Source: CAD feature listing. Evaluate the final solid. Frame: model axes, mm. A direction names the side the tool comes from. Round coordinates to 2 decimals unless told otherwise and drop trailing zeros. Write each loop counter-clockwise with the first axis right and the second up, starting at its lowest first coordinate (ties: lowest second). Pieces come first, ordered by that corner, then holes. Notation, with made-up numbers: M 67.5,77 L 93.5,77 A19 ccw 93.5,98 Z; hole C -10,13.25 d6. An arc over 180 degrees is marked long. Answer in a Markdown table with one row per item.
from build123d import *

# Parameters (mm, degrees)
STOCK_TOP_1_START                              = 44.45
STOCK_TOP_1_OUTLINE_W                          = 44.45
STOCK_TOP_1_OUTLINE_H                          = 60.96
STOCK_TOP_1_DEPTH                              = 2.54
STOCK_TOP_1_START_2                            = 43.942
STOCK_TOP_1_2_OUTLINE_W                        = 44.45
STOCK_TOP_1_2_OUTLINE_H                        = 60.96
STOCK_TOP_1_2_DEPTH                            = 0.508
OUTSIDE_FILLET_R                               = 2.54
CUT_A_BIT_OF_THE_ENCLOSURE_REACH               = 48.789
SKETCH1_W                                      = 1.334667882
SKETCH1_H                                      = 23.182275167
SKETCH2_W                                      = 3.81
SKETCH2_H                                      = 7.62
BATTERY_LID_1_DEPTH                            = 19.05
SKETCH3_W                                      = 2.54
SKETCH3_H                                      = 2.54
BATTERY_LID_HOLE_1_DEPTH                       = 1.778
CUT_EXTRUDE1_REACH                             = 64.264
SKETCH5_W                                      = 2.54
SKETCH5_H                                      = 2.54
BATTERY_LID_HOLE_2_DEPTH                       = 1.778
CUT_EXTRUDE2_REACH                             = 64.264
DETACH_LID_ATTACHEMENTS_REACH                  = 52.124
SKETCH9_W                                      = 1.524
SKETCH9_H                                      = 7.62
REMOVE_THE_INNARDS_OF_THE_LID_ATTACHMENT_DEPTH = 19.812
SKETCH11_W                                     = 1.167614697
SKETCH11_H                                     = 1.542617542
SKETCH11_W_2                                   = 1.626626063
SKETCH11_H_2                                   = 1.11023807
BOSS_EXTRUDE4_DEPTH                            = 1.778


# Read off the part's stored shape, not the designer's step: Stock-Top-1
with BuildPart() as part:
    # Stock-Top-1 outline → Stock-Top-1 (new body)
    with BuildSketch(Plane(origin=(0, 0, 0), x_dir=(1, 0, 0), z_dir=(0, 1, 0)).offset(STOCK_TOP_1_START)):
        with Locations((-1.821227893, 7.677651333)):
            Rectangle(STOCK_TOP_1_OUTLINE_W, STOCK_TOP_1_OUTLINE_H)
    extrude(amount=STOCK_TOP_1_DEPTH)

    # Stock-Top-1 2 outline → Stock-Top-1 2 (add)
    with BuildSketch(Plane(origin=(0, 0, 0), x_dir=(1, 0, 0), z_dir=(0, 1, 0)).offset(STOCK_TOP_1_START_2)):
        with Locations((-1.821227893, 7.677651333)):
            Rectangle(STOCK_TOP_1_2_OUTLINE_W, STOCK_TOP_1_2_OUTLINE_H)
        Polygon((11.494723241, -11.994444065), (17.863772107, -11.994444065), (17.863772107, -20.262348667), (-21.506227893, -20.262348667), (-21.506227893, -11.994444065), (-15.225663022, -11.994444065), (-15.225663022, 35.617651333), (11.494723241, 35.617651333), align=None, mode=Mode.SUBTRACT)
    extrude(amount=STOCK_TOP_1_2_DEPTH)

    # Enclosure: sweep along a path in Outline of Enclosure
    with BuildLine(Plane.XZ.offset(-43.942)) as enclosure_path:
        Line((-24.046227893, 22.802348667), (-24.046227893, -38.157651333))
        Line((-24.046227893, -38.157651333), (20.403772107, -38.157651333))
        Line((20.403772107, -38.157651333), (20.403772107, 22.802348667))
        Line((20.403772107, 22.802348667), (-24.046227893, 22.802348667))
    # Shape of Enclosure → Enclosure (sweep)
    with BuildSketch(Plane(origin=(20.403772107, 0, 0), x_dir=(0, 0, -1), z_dir=(1, 0, 0))):
        Polygon((38.157651333, 44.429907846), (38.442131333, 44.429907846), (38.442131333, 40.688820131), (39.070756728, 40.688820131), (39.070756728, 45.242521161), (38.157651333, 45.242521161), align=None)
    sweep(path=enclosure_path.line, transition=Transition.RIGHT)

    # Outside Fillet
    # the kernel refuses this fillet: 2.54 mm, written as the material it takes off along each edge
    with BuildSketch(Plane(origin=(20.403772107, 46.99, 28.835336218), x_dir=(2.8274047493178717e-10, -1.0, 0), z_dir=(0, 0, -1))) as outside_fillet_piece_1:
        with BuildLine():
            CenterArc((2.539999999, 2.413195021), OUTSIDE_FILLET_R, 180.000000016, 71.819221529)
            Line((-1e-09, 2.41319502), (-0.050800001, 2.41319502))
            Line((-0.050800001, 2.41319502), (-0.0508, 0))
            Line((-0.0508, 0), (0, -0.0508))
            ThreePointArc((0, -0.0508), (0.873739419, -0.0508), (1.731628415, -0.0482639))
            Line((1.731628415, -0.0482639), (1.747478839, 0))
        make_face()
    extrude(amount=73.025975102, mode=Mode.SUBTRACT)
    with BuildSketch(Plane(origin=(-24.046227893, 46.99, -44.190638886), x_dir=(2.827486071359672e-10, -1.0, 0), z_dir=(0, 0, 1))) as outside_fillet_piece_2:
        with BuildLine():
            CenterArc((2.540000001, 2.413195021), OUTSIDE_FILLET_R, 179.999999984, 71.819221529)
            Line((1e-09, 2.413195021), (-0.050799999, 2.413195021))
            Line((-0.050799999, 2.413195021), (-0.0508, 0))
            Line((-0.0508, 0), (0, -0.0508))
            ThreePointArc((0, -0.0508), (0.873739419, -0.0508), (1.731628415, -0.0482639))
            Line((1.731628415, -0.0482639), (1.747478839, 0))
        make_face()
    extrude(amount=73.025975107, mode=Mode.SUBTRACT)
    with BuildSketch(Plane(origin=(-30.079215446, 46.99, 22.802348667), x_dir=(0, -1.0, -1.349945893887387e-10), z_dir=(1, 0, 0))) as outside_fillet_piece_3:
        with BuildLine():
            CenterArc((2.54, 2.413195021), OUTSIDE_FILLET_R, 179.999999992, 71.819221529)
            Line((0, 2.413195021), (-0.0508, 2.413195021))
            Line((-0.0508, 2.413195021), (-0.0508, 0))
            Line((-0.0508, 0), (0, -0.0508))
            ThreePointArc((0, -0.0508), (0.873739419, -0.0508), (1.731628415, -0.0482639))
            Line((1.731628415, -0.0482639), (1.747478839, 0))
        make_face()
    extrude(amount=56.515975105, mode=Mode.SUBTRACT)
    with BuildSketch(Plane(origin=(26.436759659, 46.99, -38.157651333), x_dir=(0, 0, 1), z_dir=(-1, 0, 0))) as outside_fillet_piece_4:
        with BuildLine():
            CenterArc((2.413195021, -2.54), OUTSIDE_FILLET_R, 90, 71.819221529)
            Line((0, -1.747478839), (-0.048263901, -1.731628415))
            ThreePointArc((-0.048263901, -1.731628415), (-0.0508, -0.873739419), (-0.0508, 0))
            Line((-0.0508, 0), (0, 0.0508))
            Line((0, 0.0508), (2.413195021, 0.0508))
            Line((2.413195021, 0.0508), (2.413195021, 0))
        make_face()
    extrude(amount=56.515975103, mode=Mode.SUBTRACT)

    # Sketch1 → Cut a bit of the enclosure (cut, up to next)
    with BuildSketch(Plane.XZ.offset(-40.688820131), mode=Mode.PRIVATE) as cut_a_bit_of_the_enclosure_sk1:
        with Locations((-24.291999346, 12.124316479)):
            Rectangle(SKETCH1_W, SKETCH1_H)
    cut_a_bit_of_the_enclosure_tool1 = extrude(cut_a_bit_of_the_enclosure_sk1.sketch, amount=-CUT_A_BIT_OF_THE_ENCLOSURE_REACH, mode=Mode.PRIVATE) & part.part
    add(cut_a_bit_of_the_enclosure_tool1.solids().sort_by_distance((-24.291999, 40.68882, 12.124316))[0], mode=Mode.SUBTRACT)

    # Sketch2 → Battery lid 1 (add)
    with BuildSketch(Plane.XZ.offset(-43.942)):
        with Locations((-17.130663022, -8.001603634)):
            Rectangle(SKETCH2_W, SKETCH2_H)
        with Locations((13.399723241, -8.001603634)):
            Rectangle(SKETCH2_W, SKETCH2_H)
    extrude(amount=BATTERY_LID_1_DEPTH)

    # Sketch3 → Battery lid hole 1 (add)
    with BuildSketch(Plane.ZY.offset(19.035663022)):
        with Locations((-8.001603634, 37.592)):
            Rectangle(SKETCH3_W, SKETCH3_H)
    extrude(amount=BATTERY_LID_HOLE_1_DEPTH)

    # Sketch4 → Cut-Extrude1 (cut, up to next)
    with BuildSketch(Plane.XY.offset(-6.731603634), mode=Mode.PRIVATE) as cut_extrude1_sk1:
        Polygon((-20.813663022, 38.862), (-20.813663022, 36.322), (-19.924663022, 36.322), align=None)
    cut_extrude1_tool1 = extrude(cut_extrude1_sk1.sketch, amount=-CUT_EXTRUDE1_REACH, mode=Mode.PRIVATE) & part.part
    add(cut_extrude1_tool1.solids().sort_by_distance((-20.51733, 37.168667, -6.731604))[0], mode=Mode.SUBTRACT)

    # Sketch5 → Battery lid hole 2 (add)
    with BuildSketch(Plane(origin=(15.304723241, 0, 0), x_dir=(0, 0, -1), z_dir=(1, 0, 0))):
        with Locations((8.001603634, 37.592)):
            Rectangle(SKETCH5_W, SKETCH5_H)
    extrude(amount=BATTERY_LID_HOLE_2_DEPTH)

    # Sketch6 → Cut-Extrude2 (cut, up to next)
    with BuildSketch(Plane.XY.offset(-6.731603634), mode=Mode.PRIVATE) as cut_extrude2_sk1:
        Polygon((17.082723241, 38.862), (17.082723241, 36.322), (15.812723241, 36.322), align=None)
    cut_extrude2_tool1 = extrude(cut_extrude2_sk1.sketch, amount=-CUT_EXTRUDE2_REACH, mode=Mode.PRIVATE) & part.part
    add(cut_extrude2_tool1.solids().sort_by_distance((16.65939, 37.168667, -6.731604))[0], mode=Mode.SUBTRACT)

    # Sketch7 → Detach Lid attachements (cut, up to next)
    with BuildSketch(Plane.XZ.offset(-43.942), mode=Mode.PRIVATE) as detach_lid_attachements_sk1:
        Polygon((-16.469097924, -4.191603634), (-19.035663022, -4.191603634), (-19.035663022, -6.731603634), (-21.429165636, -6.731603634), (-21.429165636, -9.410456582), (-19.035663022, -9.410456582), (-19.035663022, -11.811603634), (-16.469097924, -11.811603634), (-16.469097924, -12.285051826), (-19.771097924, -12.285051826), (-19.771097924, -9.817750336), (-22.345673393, -9.817750336), (-22.345673393, -6.870456582), (-22.345673393, -6.492257022), (-19.771097924, -6.492257022), (-19.771097924, -3.953439546), (-16.469097924, -3.953439546), align=None)
    detach_lid_attachements_tool1 = extrude(detach_lid_attachements_sk1.sketch, amount=-DETACH_LID_ATTACHEMENTS_REACH, mode=Mode.PRIVATE) & part.part
    # Sketch7 → Detach Lid attachements (cut, up to next)
    with BuildSketch(Plane.XZ.offset(-43.942), mode=Mode.PRIVATE) as detach_lid_attachements_sk2:
        Polygon((12.764723241, -4.191603634), (15.304723241, -4.191603634), (15.304723241, -6.731603634), (17.082723241, -6.731603634), (17.082723241, -9.271603634), (15.304723241, -9.271603634), (15.304723241, -11.811603634), (12.764723241, -11.811603634), (12.764723241, -12.319603634), (15.812723241, -12.319603634), (15.812723241, -9.624506021), (18.02600878, -9.624506021), (18.02600878, -6.09262067), (15.685723241, -6.09262067), (15.685723241, -3.683603634), (12.764723241, -3.683603634), align=None)
    detach_lid_attachements_tool2 = extrude(detach_lid_attachements_sk2.sketch, amount=-DETACH_LID_ATTACHEMENTS_REACH, mode=Mode.PRIVATE) & part.part
    add(detach_lid_attachements_tool1.solids().sort_by_distance((-17.75238, 43.942, -4.089648))[0], mode=Mode.SUBTRACT)
    add(detach_lid_attachements_tool2.solids().sort_by_distance((14.034723, 43.942, -4.090479))[0], mode=Mode.SUBTRACT)

    # Sketch9 → Remove the innards of the lid attachment (cut)
    with BuildSketch(Plane(origin=(0, 46.99, 0), x_dir=(1, 0, 0), z_dir=(0, 1, 0))):
        with Locations((-17.257663022, 8.001603634)):
            Rectangle(SKETCH9_W, SKETCH9_H)
        with Locations((13.526723241, 8.001603634)):
            Rectangle(SKETCH9_W, SKETCH9_H)
    extrude(amount=-REMOVE_THE_INNARDS_OF_THE_LID_ATTACHMENT_DEPTH, mode=Mode.SUBTRACT)

    # Sketch11 → Boss-Extrude4 (add)
    with BuildSketch(Plane(origin=(0, 46.99, 0), x_dir=(1, 0, 0), z_dir=(0, 1, 0))):
        with Locations((15.362507718, 8.090206817)):
            Rectangle(SKETCH11_W, SKETCH11_H)
        with Locations((-19.754773261, 8.124447803)):
            Rectangle(SKETCH11_W_2, SKETCH11_H_2)
    extrude(amount=BOSS_EXTRUDE4_DEPTH)


solid = part.part
Q1. Section A-A (y = 41.75). Return loops of the section in (x, z).
Solutions:
| item | result |
|---|---|
| outline | M -24.96,-39.07 L 21.32,-39.07 L 21.32,23.72 L -23.62,23.72 L -23.62,23.09 L 20.69,23.09 L 20.69,-38.44 L -24.33,-38.44 L -24.33,0.53 L -24.96,0.53 Z; M -19.04,-11.81 L -18.02,-11.81 L -18.02,-4.19 L -19.04,-4.19 Z; M -16.5,-11.81 L -15.23,-11.81 L -15.23,-4.19 L -16.5,-4.19 Z; M 11.49,-11.81 L 12.76,-11.81 L 12.76,-4.19 L 11.49,-4.19 Z; M 14.29,-11.81 L 15.3,-11.81 L 15.3,-4.19 L 14.29,-4.19 Z |
Q2. Section D-D (z = 16.5). Return loops of the section in (x, y).
Solutions:
| item | result |
|---|---|
| outline | M -23.62,43.94 L -21.51,43.94 L -21.51,44.45 L 17.86,44.45 L 17.86,43.94 L 20.4,43.94 L 20.4,44.43 L 20.69,44.43 L 20.69,40.69 L 21.32,40.69 L 21.32,45.24 L 20.4,45.24 A2.54 ccw 17.99,46.99 L -21.63,46.99 A2.54 ccw -23.62,46.03 Z |
Q3. Pull-direction query (Z, two-part tool) for faces 6 (the flat face through (-21, 45, -6.492)), 7 (the flat face through (-20.36, 37.57, -7.98)), 8 (the cylindrical face through (-1.92, 46.52, 21.86)); classes: pulls with the +Z half, pulls with the -Z half, needs draft (parallel to the pull), parting line crosses it, or undercut.
Solutions:
| item | result |
|---|---|
| face 6 | undercut |
| face 7 | needs draft |
| face 8 | pulls with the +Z half |
Q4. Section B-B (y = 33). Return loops of the section in (x, z).
Solutions:
| item | result |
|---|---|
| outline | M -19.04,-11.81 L -18.02,-11.81 L -18.02,-4.19 L -19.04,-4.19 Z; M -16.5,-11.81 L -15.23,-11.81 L -15.23,-4.19 L -16.5,-4.19 Z; M 11.49,-11.81 L 12.76,-11.81 L 12.76,-4.19 L 11.49,-4.19 Z; M 14.29,-11.81 L 15.3,-11.81 L 15.3,-4.19 L 14.29,-4.19 Z |
Q5. Contact query for flat-ended pins moving along their axis: pin 1 Ø0.6 at (x, y) = (15.5, 48) entering from -Z; pin 2 Ø3 at (x, z) = (-7, -9.5) entering from -Y; pin 3 Ø2 at (x, y) = (-19, 36.5) entering from -Z; pin 4 Ø5 at (y, z) = (36.5, -17.5) entering from -X. Output: stop coordinate, or through.
Solutions:
| item | result |
|---|---|
| pin 1 | stops at z = -8.86 |
| pin 2 | stops at y = 44.45 |
| pin 3 | stops at z = -11.81 |
| pin 4 | passes through |
Q6. Section C-C (x = 5). Return loops of the section in (y, z).
Solutions:
| item | result |
|---|---|
| outline | M 40.69,-39.07 L 45.24,-39.07 L 45.24,-38.16 A2.54 ccw 46.99,-35.74 L 46.99,20.39 A2.54 ccw 45.24,22.8 L 45.24,23.72 L 40.69,23.72 L 40.69,23.09 L 44.43,23.09 L 44.43,22.8 L 43.94,22.8 L 43.94,20.26 L 44.45,20.26 L 44.45,-35.62 L 43.94,-35.62 L 43.94,-38.16 L 44.43,-38.16 L 44.43,-38.44 L 40.69,-38.44 Z |
Q7. Material intervals for probe 1 along X at (y, z) = (40, -6.5); probe 2 along Z at (x, y) = (-7, 44.25); probe 3 along Z at (x, y) = (-13.5, 41.25), sorted ascending.
Solutions:
| item | result |
|---|---|
| probe 1 | x = -19.04 to -18.02, -16.5 to -15.23, 11.49 to 12.76, 14.29 to 15.3 |
| probe 2 | z = -39.07 to -38.44, -38.16 to -35.62, 20.26 to 22.8, 23.09 to 23.72 |
| probe 3 | z = -39.07 to -38.44, 23.09 to 23.72 |
Q8. Access query for faces 1 (the flat face through (-17, 27.178, -8)), 2 (the flat face through (15.946, 48, -8)), 3 (the flat face through (-16, 34, -11.812)), 4 (the flat face through (14, 45, -12.32)), 5 (the flat face through (-20, 38, -6.732)). Directions: +Z, -Z, +X, -X, +Y, -Y. A direction counts if a zero-diameter tool reaches every point of the face in a straight line with its end or side. Return the directions, or none.
Solutions:
| item | result |
|---|---|
| face 1 | +Z, -Z, +Y |
| face 2 | +Z, -Z, +X, +Y |
| face 3 | -Y |
| face 4 | +Y, -Y |
| face 5 | +Z, -X, +Y, -Y |
